Part model, mm, in its own coordinate system. A direction names the side the tool comes from. Round coordinates to 2 decimals unless told otherwise and drop trailing zeros. Loops run counter-clockwise (first coordinate to the right, second up) from the corner with the lowest first, then second, coordinate; pieces in that order, holes last. Notation, with made-up numbers: M 48.25,-1.5 L 79.25,-1.5 A7 ccw 79.25,9.5 Z; hole C -30,-39.5 d6. An arc over 180 degrees is marked long. Answer as CSV lines item,"result". Start each with the question number.
Item 1: Band-saw the part on C-C (z = 4.25). Count the separate pieces of the cut face and the enclosed holes in it, and give its area (3 significant figures).
Item 2: Drop a flat-ended pin along its axis: pin 1 Ø4 at (x, z) = (83.5, 6.5) entering from -Y. Give the stop position or say it passes through.
Item 3: Band-saw the part on B-B (y = -76). Give the cut face in (x, z), and give its area (3 significant figures).
Item 4: Band-saw the part on D-D (x = 21.2). Give the cut face in (y, z).
Item 5: Which spindle directions (+Z, -Z, +X, -X, +Y, -Y) get a long thin tool onto all of the face, cutting with end or side? Do faces 1 (the flat face through (75, -60, 4)), 2 (the cylindrical face through (10.536, -9.061, 4.056)). Say none if no direction does.
Item 6: Band-saw the part on A-A (x = 42). Give the cut face in (y, z).
Item 7: Wall check: line 1 (X direction, y = -29.5, z = 1.25); line 2 (Y direction, x = 59.5, z = 0.5); line 3 (Y direction, x = 9, z = 5.75). Give the ranges that are in metal, low to high.
```python
from build123d import *

# Parameters (mm, degrees)
SKETCH_1_R          = 2.75
SKETCH_1_R_2        = 14
SKETCH_1_R_3        = 11.5
SKETCH_1_R_4        = 2
EXTRUDE_1_DEPTH     = 8
FILLET_1_R          = 5
SKETCH_2_R          = 2.3
CUT_EXTRUDE_1_DEPTH = 10


with BuildPart() as part:
    # 草图1 → 凸台-拉伸1 (new body)
    with BuildSketch(Plane.XY):
        Polygon((0, 0), (54, 0), (96, 0), (96, -60), (54, -60), (54, -110), (0, -110), align=None)
        with Locations((12, -106)):
            Circle(SKETCH_1_R, mode=Mode.SUBTRACT)
        with Locations((42, -106)):
            Circle(SKETCH_1_R, mode=Mode.SUBTRACT)
        with Locations((42, -76)):
            Circle(SKETCH_1_R, mode=Mode.SUBTRACT)
        with Locations((12, -76)):
            Circle(SKETCH_1_R, mode=Mode.SUBTRACT)
        with Locations((21.2, -30)):
            Circle(SKETCH_1_R_2, mode=Mode.SUBTRACT)
        with Locations((74.7, -30)):
            Circle(SKETCH_1_R_3, mode=Mode.SUBTRACT)
        with Locations((59.2, -14.5)):
            Circle(SKETCH_1_R_4, mode=Mode.SUBTRACT)
        with Locations((90.2, -14.5)):
            Circle(SKETCH_1_R_4, mode=Mode.SUBTRACT)
        with Locations((90.2, -45.5)):
            Circle(SKETCH_1_R_4, mode=Mode.SUBTRACT)
        with Locations((59.2, -45.5)):
            Circle(SKETCH_1_R_4, mode=Mode.SUBTRACT)
    extrude(amount=EXTRUDE_1_DEPTH)

    # 圆角1
    fillet_1_edges = [part.edges().sort_by_distance(p)[0] for p in [
        (0, 0, 4),
        (96, 0, 4),
        (96, -60, 4),
        (54, -60, 4),
    ]]
    fillet(fillet_1_edges, radius=FILLET_1_R)

    # 草图2 → 切除-拉伸1 (cut)
    with BuildSketch(Plane.XY.offset(8)):
        with Locations((9.3, -11)):
            Circle(SKETCH_2_R)
        with Locations((33.3, -11)):
            Circle(SKETCH_2_R)
        with Locations((33.3, -49)):
            Circle(SKETCH_2_R)
        with Locations((9.3, -49)):
            Circle(SKETCH_2_R)
    extrude(amount=-CUT_EXTRUDE_1_DEPTH, mode=Mode.SUBTRACT)


solid = part.part
```
Answer block:
1,separate pieces,"1"
1,enclosed holes,"14"
1,area,"7,210 mm^2"
2,pin 1,"stops at y = -60"
3,outline,"M 0,0 L 9.25,0 L 9.25,8 L 0,8 Z; M 14.75,0 L 39.25,0 L 39.25,8 L 14.75,8 Z; M 44.75,0 L 54,0 L 54,8 L 44.75,8 Z"
3,area,"344 mm^2"
4,outline,"M -110,0 L -44,0 L -44,8 L -110,8 Z; M -16,0 L 0,0 L 0,8 L -16,8 Z"
5,face 1,"+Z, -Z, +X, -Y"
5,face 2,"+Z, -Z"
6,outline,"M -110,0 L -108.75,0 L -108.75,8 L -110,8 Z; M -103.25,0 L -78.75,0 L -78.75,8 L -103.25,8 Z; M -73.25,0 L 0,0 L 0,8 L -73.25,8 Z"
7,line 1,"x = 0 to 7.21, 35.19 to 63.21, 86.19 to 96"
7,line 2,"y = -60 to -47.48, -43.52 to -16.48, -12.52 to 0"
7,line 3,"y = -110 to -51.28, -46.72 to -36.87, -23.13 to -13.28, -8.72 to 0"
